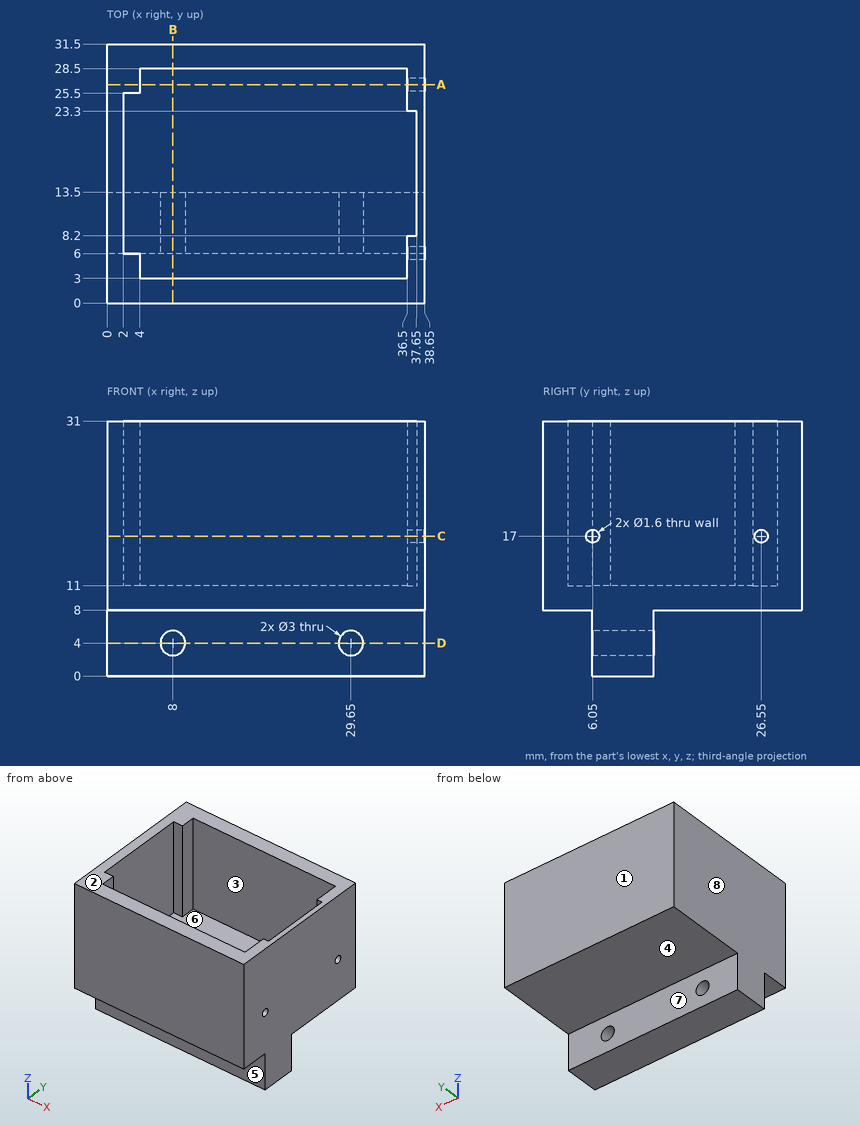
Source: three-view drawing plus pictorial views. Frame: mm from the lowest corner of the part. A direction names the side the tool comes from. Give positions to 0.01 mm unless a question says otherwise; leave off trailing zeros. Order: outer loops, then holes, each group sorted by start corner. A loop starts at its lowest first (then second) coordinate and runs counter-clockwise, first axis right, second up. Notation, with made-up numbers: (6.5, -6) - (61.5, -6) arc R6 ccw to (61.5, 1) - close; hole circle Ø5 at (-24.75, 28.5). An arc over 180 degrees is marked (long way). Answer as a JSON object with one key per item and string values. Group by question number.
Q1. Mould query, pull axis Y, two halves, no side actions, for the marked faces 6, 7 and 8. Classes: pulls with the +Y half, pulls with the -Y half, needs draft (parallel to the pull), parting line crosses it, or undercut.
Q2. Set-up query: the marked faces 1, 2, 3, 4 and 5. Return all of +Z, -Z, +X, -X, +Y, -Y with unobstructed straight access to the full face (end or side cutting, diameter ignored); none if empty.
Q3. Cut plane C-C, the plane z = 17. Output: boundary loops of the cut face in (x, y).
Q4. Cut plane D-D, the plane z = 4. Output: boundary loops of the cut face in (x, y).
Q5. Line query: probe 1 along X at (y, z) = (9, 4); probe 2 along Y at (x, z) = (37.5, 17); probe 3 along Y at (x, z) = (34, 27.5). Output: solid intervals per line, ascending.
Q6. Cut plane B-B, the plane x = 8. Output: boundary loops of the cut face in (y, z).
Q7. First-contact query: pin 1 Ø5 at (x, z) = (29.65, 4) entering from -Y; pin 2 Ø7.5 at (x, y) = (15, 13.5) entering from +Z; pin 3 Ø5.5 at (x, y) = (12, 22) entering from -Z. Flat tips, straight axial feed; report the tip coordinate or a pass-through.
Q8. Cut plane A-A, the plane y = 26.55. Output: boundary loops of the cut face in (x, z), then the cut area to 3 significant figures.
Results:
{
 "1": {"face 6": "undercut", "face 7": "pulls with the +Y half", "face 8": "needs draft"},
 "2": {"face 1": "+Z, -Z, +X, -X, +Y", "face 2": "+Z, +X, -X, +Y, -Y", "face 3": "+Z", "face 4": "-Z, +X, -X, +Y", "face 5": "-Z, +X, -X, -Y"},
 "3": {"outline": "(0, 0) - (38.65, 0) - (38.65, 5.25) - (36.5, 5.25) - (36.5, 3) - (4, 3) - (4, 6) - (2, 6) - (2, 25.5) - (4, 25.5) - (4, 28.5) - (36.5, 28.5) - (36.5, 27.35) - (38.65, 27.35) - (38.65, 31.5) - (0, 31.5) - close; (36.5, 6.85) - (38.65, 6.85) - (38.65, 25.75) - (36.5, 25.75) - (36.5, 23.3) - (37.65, 23.3) - (37.65, 8.2) - (36.5, 8.2) - close"},
 "4": {"outline": "(0, 6) - (6.5, 6) - (6.5, 13.5) - (0, 13.5) - close; (9.5, 6) - (28.15, 6) - (28.15, 13.5) - (9.5, 13.5) - close; (31.15, 6) - (38.65, 6) - (38.65, 13.5) - (31.15, 13.5) - close"},
 "5": {"probe 1": "0 to 6.5, 9.5 to 28.15, 31.15 to 38.65", "probe 2": "0 to 5.25, 6.85 to 8.2, 23.3 to 25.75, 27.35 to 31.5", "probe 3": "0 to 3, 28.5 to 31.5"},
 "6": {"outline": "(0, 8) - (6, 8) - (6, 5.5) - (13.5, 5.5) - (13.5, 8) - (31.5, 8) - (31.5, 31) - (28.5, 31) - (28.5, 11) - (3, 11) - (3, 31) - (0, 31) - close; (6, 0) - (13.5, 0) - (13.5, 2.5) - (6, 2.5) - close"},
 "7": {"pin 1": "y = 6", "pin 2": "z = 11", "pin 3": "z = 8"},
 "8": {"outline": "(0, 8) - (38.65, 8) - (38.65, 16.2) - (36.5, 16.2) - (36.5, 11) - (4, 11) - (4, 31) - (0, 31) - close; (36.5, 17.8) - (38.65, 17.8) - (38.65, 31) - (36.5, 31) - close", "area": "236 mm^2"}
}
